The listing builds one solid part. Answer for the finished solid, in the listing's coordinates (mm). A direction names the side the tool comes from. Round coordinates to 2 decimals unless told otherwise and drop trailing zeros. Order: outer loops, then holes, each group sorted by start corner. A loop starts at its lowest first (then second) coordinate and runs counter-clockwise, first axis right, second up. Notation, with made-up numbers: (5.25, -33) - (11.25, -33) arc R27 ccw to (11.25, -6) - close; hole circle Ø5 at (-9, 63). An arc over 180 degrees is marked (long way). Write item = value, one per line.
from build123d import *

# Parameters (mm, degrees)
F0_W     = 10
F0_H     = 38.9
F1_DEPTH = 3
F0_H_2   = 5.6
F0_R     = 1.25
F2_DEPTH = 6


with BuildPart() as f1:
    # F0 (on Top) → F1 (new body)
    with BuildSketch(Plane.XY):
        Rectangle(F0_W, F0_H)
    extrude(amount=F1_DEPTH)

    # F0 (on Top) → F2 (join)
    with BuildSketch(Plane.XY):
        with Locations((0, 22.25)):
            Rectangle(F0_W, F0_H_2)
        with Locations((-2.75, 22.25)):
            Circle(F0_R, mode=Mode.SUBTRACT)
        with Locations((2.75, 22.25)):
            Circle(F0_R, mode=Mode.SUBTRACT)
        with Locations((0, -22.25)):
            Rectangle(F0_W, F0_H_2)
        with Locations((-2.75, -22.25)):
            Circle(F0_R, mode=Mode.SUBTRACT)
        with Locations((2.75, -22.25)):
            Circle(F0_R, mode=Mode.SUBTRACT)
    extrude(amount=F2_DEPTH)


solid = f1.part
Q1. Find the intervals of material crossed by line 1 (Y direction, x = 2.75, z = 1.7); line 2 (Y direction, x = -2.75, z = 4.8); line 3 (Y direction, x = 1, z = 3.45), in increasing order. Write a range as from..to.
Model answer:
line_1 = -25.05..-23.5, -21..21, 23.5..25.05
line_2 = -25.05..-23.5, -21..-19.45, 19.45..21, 23.5..25.05
line_3 = -25.05..-19.45, 19.45..25.05
Q2. For faces 4 (the face through (-3.02, 21.03, 2.96)), 5 (the face through (0, 19.45, 4)), determine the directions among +Z, -Z, +X, -X, +Y, -Y from which every point of the face is accessible in a straight line to the end or side of a thin tool.
Model answer:
face_4 = +Z, -Z
face_5 = +Z, +X, -X
Q3. Section D-D on z = 0.95 is taken. Determine the outline of the cut face in (x, y), then the cut area to 3 significant figures.
Model answer:
outline = (-5, -25.05) - (5, -25.05) - (5, 25.05) - (-5, 25.05) - close; hole circle Ø2.5 at (-2.75, -22.25); hole circle Ø2.5 at (-2.75, 22.25); hole circle Ø2.5 at (2.75, -22.25); hole circle Ø2.5 at (2.75, 22.25)
area = 481 mm^2
Q4. Flat-ended cylindrical pins translate along their axes: P1, Ø5, axis at x = 1.5, y = 5.5, coming from the -Z side; P2, Ø2, axis at x = -3.5, y = 12.5, coming from the +Z side. Find the tip coordinate at first contact, or state that the pin passes through.
Model answer:
P1 = 0
P2 = 3
Q5. Section A-A on z = 5 is taken. Determine the outline of the cut face in (x, y).
Model answer:
outline = (-5, -25.05) - (5, -25.05) - (5, -19.45) - (-5, -19.45) - close; (-5, 19.45) - (5, 19.45) - (5, 25.05) - (-5, 25.05) - close; hole circle Ø2.5 at (-2.75, -22.25); hole circle Ø2.5 at (-2.75, 22.25); hole circle Ø2.5 at (2.75, -22.25); hole circle Ø2.5 at (2.75, 22.25)
Q6. Section C-C on x = -2.75 is taken. Determine the outline of the cut face in (y, z).
Model answer:
outline = (-25.05, 0) - (-23.5, 0) - (-23.5, 6) - (-25.05, 6) - close; (-21, 0) - (21, 0) - (21, 6) - (19.45, 6) - (19.45, 3) - (-19.45, 3) - (-19.45, 6) - (-21, 6) - close; (23.5, 0) - (25.05, 0) - (25.05, 6) - (23.5, 6) - close
Q7. Section B-B on y = -22.25 is taken. Determine the outline of the cut face in (x, z).
Model answer:
outline = (-5, 0) - (-4, 0) - (-4, 6) - (-5, 6) - close; (-1.5, 0) - (1.5, 0) - (1.5, 6) - (-1.5, 6) - close; (4, 0) - (5, 0) - (5, 6) - (4, 6) - close
Q8. Determine the mould class of faces 1 (the face through (0, 25.05, 3)), 2 (the face through (-3.02, -23.47, 2.96)), 3 (the face through (0, 22, 6)) for opening direction Y: released by +Y, released by -Y, zero draft, split by the parting line, or undercut.
Model answer:
face_1 = released by +Y
face_2 = undercut
face_3 = zero draft
